Build history of the part. All positions in model axes, mm. Face numbers are marked on the shaded views. A direction names the side the tool comes from. Coordinates: 2 decimals unless noted, no trailing zeros. Order: outer loops, then holes, each group sorted by start corner. A loop starts at its lowest first (then second) coordinate and runs counter-clockwise, first axis right, second up. Notation, with made-up numbers: M -24,30 L 14,30 A34 ccw 14,68 Z; hole C 41,61 d11. An arc over 180 degrees is marked long. Write item = value, one per line. Start each with the question number.
Q1. Pin check, flat tips, straight feed: P1, Ø1, axis at y = 3, z = 17, coming from the -X side; P2, Ø2.5, axis at x = 0, y = 0, coming from the -Z side; P3, Ø1.5, axis at x = 2, y = 2.5, coming from the -Z side; P4, Ø1.5, axis at x = -0.5, y = 0, coming from the +Z side. Stop position of each tip, or through.
Q2. Drill centre lines: probe 1 along Y at (x, z) = (0, 22); probe 2 along Z at (x, y) = (1.25, 0.25); probe 3 along Y at (x, z) = (-1, 22.75). Where is each one in solid material? Low to high.
Q3. Band-saw the part on A-A on x = 0. Write the cut outline in (y, z).
Q4. Band-saw the part on D-D on z = 23.5. Write the cut outline in (x, y).
Q5. Band-saw the part on C-C on z = 16. Write the cut outline in (x, y).
Q6. 3-axis set-ups, long thin cutter, end or side, ignore diameter. For the marked faces 4 and 5: which of +Z, -Z, +X, -X, +Y, -Y reach the whole face in a straight line?
Q7. Pull direction Y, two halves, no side cores. Call the marked faces 1, 2 and 3: released by +Y, released by -Y, zero draft, split by the parting line, or undercut.
Autodesk Fusion 360 part; units mm, degrees
sketch "スケッチ1" plane through (0, 0, 0) normal (0, 0, 1) x (1, 0, 0)
  circle A0 centre (0, 0) radius 4
  dimension "d1" = 8
extrude "押し出し1" add sketch "スケッチ1" along normal blind 25
cylinder "円柱プリミティブ2" cut diameter 3 height -5 placed x (1, 0, 0) y (0, 1, 0) z (0, 0, 1) at (0, 0, 25)
thread "ねじ2" thread offset 0 thread length 10
cylinder "円柱プリミティブ3" cut diameter 3 height -5 placed x (0, 1, 0) y (1, 0, 0) z (0, 0, -1) at (0, 0, 0)
thread "ねじ3" thread offset 0 thread length 10
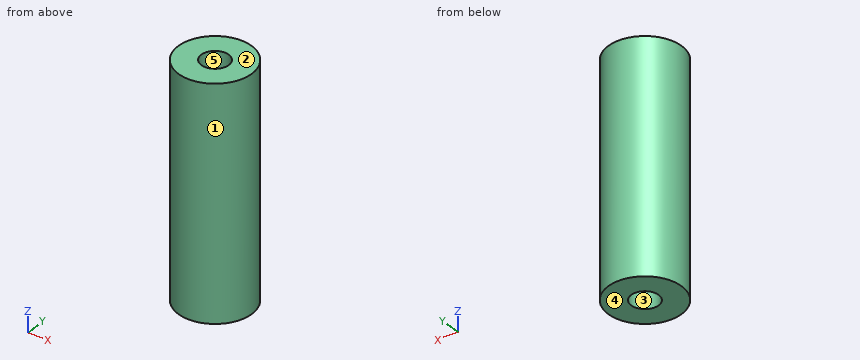
Recorded:
q1.P1 = -3.12
q1.P2 = 5
q1.P3 = 0
q1.P4 = 20
q2.probe_1 = -4 to -1.5, 1.5 to 4
q2.probe_2 = 5 to 20
q2.probe_3 = -3.87 to -1.12, 1.12 to 3.87
q3.outline = M -4,0 L -1.5,0 L -1.5,5 L 1.5,5 L 1.5,0 L 4,0 L 4,25 L 1.5,25 L 1.5,20 L -1.5,20 L -1.5,25 L -4,25 Z
q4.outline = C 0,0 d8; hole C 0,0 d3
q5.outline = C 0,0 d8
q6.face_4 = -Z, +X, -X, +Y, -Y
q6.face_5 = +Z
q7.face_1 = split by the parting line
q7.face_2 = zero draft
q7.face_3 = undercut
